Part model, mm, in its own coordinate system. Coordinates: 2 decimals unless noted, no trailing zeros. Order: outer loops, then holes, each group sorted by start corner. A loop starts at its lowest first (then second) coordinate and runs counter-clockwise, first axis right, second up.
1) Cut at D-D (x = -5). List the corners of the cut face in (y, z), and give its area (3 significant figures).
2) Mould opens along Y. For faces 1 (the flat face through (70, 4, 4)), 2 (the cylindrical face through (11.7, -4.88, 1.08)), 3 (the cylindrical face through (12, 0, 6)) say: +Y half, -Y half, draft (parallel to the pull), parting line (faces both ways), or undercut.
3) Pin check, flat tip, straight feed: pin 1 Ø3 at (x, z) = (-35, 0) entering from -Y. Stop position of the tip, or through.
4) Cut at C-C (x = 35). List the corners of the cut face in (y, z).
5) Cut at A-A (y = 0). List the corners of the cut face in (x, z), and give its area (3 significant figures).
6) Cut at B-B (z = 0). Give the number of separate pieces and of enclosed holes in the cut face, and give its area (3 significant figures).
7) Wall check: L1, parallel to X at y = 5.15, z = 0; L2, parallel to Y at x = -39, z = -0.25. Give the ranges that are in metal, low to high.
```python
from build123d import *

# Parameters (mm, degrees)
SKETCH1_R           = 6
SKETCH1_R_2         = 5
BOSS_EXTRUDE1_DEPTH = 45
SKETCH3_R           = 6
SKETCH3_R_2         = 5
BOSS_EXTRUDE2_DEPTH = 25
SKETCH2_R           = 2
CUT_EXTRUDE1_DEPTH  = 10


with BuildPart() as part:
    # Sketch1 → Boss-Extrude1 (new body, symmetric)
    with BuildSketch(Plane(origin=(0, 0, 0), x_dir=(0, 0, -1), z_dir=(1, 0, 0))):
        Circle(SKETCH1_R)
        Circle(SKETCH1_R_2, mode=Mode.SUBTRACT)
    extrude(amount=BOSS_EXTRUDE1_DEPTH, both=True)

    # Sketch3 → Boss-Extrude2 (add)
    with BuildSketch(Plane(origin=(45, 0, 0), x_dir=(0, 0, -1), z_dir=(1, 0, 0))):
        Circle(SKETCH3_R)
        Circle(SKETCH3_R_2, mode=Mode.SUBTRACT)
    extrude(amount=BOSS_EXTRUDE2_DEPTH)

    # Sketch2 → Cut-Extrude1 (cut, symmetric)
    with BuildSketch(Plane(origin=(0, 0, 0), x_dir=(1, 0, 0), z_dir=(0, 1, 0))):
        with Locations((-35, 0)):
            Circle(SKETCH2_R)
        with Locations((35, 0)):
            Circle(SKETCH2_R)
        with Locations((60, 0)):
            Circle(SKETCH2_R)
    extrude(amount=CUT_EXTRUDE1_DEPTH, both=True, mode=Mode.SUBTRACT)


solid = part.part
```
Geometry check:
1. outline: circle Ø12 at (0, 0); hole circle Ø10 at (0, 0)
1. area: 34.6 mm2
2. face 1: draft
2. face 2: undercut
2. face 3: parting line
3. pin 1: passes through
4. outline: (-5.66, -2) arc R6 ccw to (5.66, -2) - (4.58, -2) arc R5 cw to (-4.58, -2) - close; (-5.66, 2) - (-4.58, 2) arc R5 cw to (4.58, 2) - (5.66, 2) arc R6 ccw to start
5. outline: (-45, -6) - (70, -6) - (70, -5) - (-45, -5) - close; (-45, 5) - (70, 5) - (70, 6) - (-45, 6) - close
5. area: 230 mm2
6. separate pieces: 8
6. enclosed holes: 0
6. area: 206 mm2
7. L1: x = -45 to -37, -33 to 33, 37 to 58, 62 to 70
7. L2: y = -5.99 to -4.99, 4.99 to 5.99
